Study the drawing (mm; zero at the part's minimum x, y, z) and answer. A direction names the side the tool comes from. Coordinates: 2 decimals unless noted, no trailing zeros. Order: outer loops, then holes, each group sorted by start corner. A loop starts at its lowest first (then second) coordinate and runs counter-clockwise, first axis right, second up.
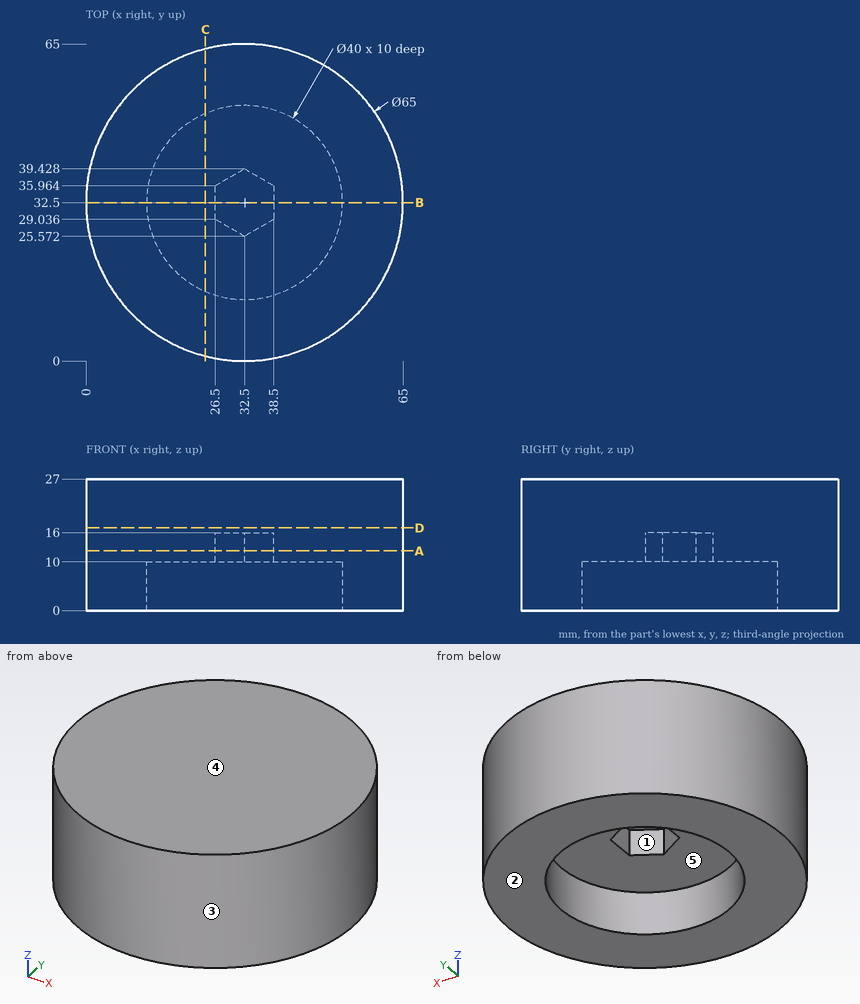
1) A cutting plane is placed at D-D, the plane z = 17. Determine the outline of the cut face in (x, y), and give its area (3 significant figures).
A:
outline: circle Ø65 at (32.5, 32.5)
area: 3,320 mm2
2) A cutting plane is placed at C-C, the plane x = 24.5. Determine the outline of the cut face in (y, z), and give its area (3 significant figures).
A:
outline: (1, 0) - (14.17, 0) - (14.17, 10) - (50.83, 10) - (50.83, 0) - (64, 0) - (64, 27) - (1, 27) - close
area: 1,330 mm2
3) Flat-ended cylindrical pins translate along their axes: pin 1 Ø1 at (y, z) = (11.5, 23.5) entering from +X; pin 2 Ø6 at (x, y) = (35, 32) entering from -Z; pin 3 Ø3 at (y, z) = (55, 20) entering from -X. Find the tip coordinate at first contact, or state that the pin passes through.
A:
pin 1: stops at x = 57.72
pin 2: stops at z = 16
pin 3: stops at x = 7.7
4) A cutting plane is placed at A-A, the plane z = 12.25. Determine the outline of the cut face in (x, y), and give its area (3 significant figures).
A:
outline: circle Ø65 at (32.5, 32.5); hole (26.5, 29.04) - (32.5, 25.57) - (38.5, 29.04) - (38.5, 35.96) - (32.5, 39.43) - (26.5, 35.96) - close
area: 3,190 mm2
5) Straight lines are drawn through the part: line 1 (Y direction, x = 32.5, z = 4.5); line 2 (Z direction, x = 45.5, y = 42.5); line 3 (Y direction, x = 29, z = 19). For each, find the intervals that lie inside material, in ascending order.
A:
line 1: y = 0 to 12.5, 52.5 to 65
line 2: z = 10 to 27
line 3: y = 0.19 to 64.81
6) A cutting plane is placed at B-B, the plane y = 32.5. Determine the outline of the cut face in (x, z), and give its area (3 significant figures).
A:
outline: (0, 0) - (12.5, 0) - (12.5, 10) - (26.5, 10) - (26.5, 16) - (38.5, 16) - (38.5, 10) - (52.5, 10) - (52.5, 0) - (65, 0) - (65, 27) - (0, 27) - close
area: 1,280 mm2
7) Determine the mould class of the marked faces 3, 4 and 5 for opening direction Y: pulls with the +Y half, pulls with the -Y half, needs draft (parallel to the pull), parting line crosses it, or undercut.
A:
face 3: parting line crosses it
face 4: needs draft
face 5: undercut
8) Which of the six approach directions +Z, -Z, +X, -X, +Y, -Y give full straight-line access (tool end or side, diameter ignored) to the marked faces 1 and 2?
A:
face 1: -Z
face 2: -Z, +X, -X, +Y, -Y
